The listing builds one solid part. Answer for the finished solid, in the listing's coordinates (mm). Round coordinates to 2 decimals unless told otherwise and drop trailing zeros. Order: outer loops, then holes, each group sorted by start corner. A loop starts at its lowest first (then second) coordinate and runs counter-clockwise, first axis right, second up. Notation, with made-up numbers: (-34, 33) - (0, 33) arc R28 ccw to (0, 70) - close; hole circle Ø8 at (47.25, -19.5). An arc over 180 degrees is marked (long way). One line per item, written item: value. Start each with the question number.
1. Section B-B, the plane y = 0 is taken. Give the vertices of the cut face in (x, z).
2. Section A-A, the plane z = 6.5 is taken. Give the vertices of the cut face in (x, y).
3. Straight lines are drawn through the part: line 1 (Z direction, x = -1.75, y = 1.6); line 2 (Z direction, x = 8, y = -2.55); line 3 (X direction, y = 0, z = 3.5). For each, find the intervals that lie inside material, in ascending order.
4. Flat-ended cylindrical pins translate along their axes: P1, Ø3.5, axis at x = 8, z = 33.5, coming from the -Y side; P2, Ø1.5, axis at y = -2, z = 8.5, coming from the -X side; P3, Ø0.5, axis at y = -2, z = 27.5, coming from the -X side; P4, Ø2.5, axis at x = 8, z = 6.5, coming from the +Y side. Find the tip coordinate at first contact, or state that the pin passes through.
5. Section D-D, the plane z = 21.5 is taken. Give the vertices of the cut face in (x, y), then the cut area to 3 significant figures.
6. Section C-C, the plane x = 8 is taken. Give the vertices of the cut face in (y, z).
from build123d import *

# Parameters (mm, degrees)
ESQUISSE1_R                  = 1.75
BOSS_EXTRU_1_DEPTH           = 40
ENL_V_MAT_EXTRU_3_DEPTH      = 20
ENL_V_MAT_EXTRU_3_DEPTH_BACK = 20
ESQUISSE2_W                  = 17.8
ESQUISSE2_H                  = 8
D_GAGEMENT_M31_D             = 3
D_GAGEMENT_M31_DEPTH         = 10
D_GAGEMENT_M31_CSINK_D       = 4.4
D_GAGEMENT_M31_CSINK_ANGLE   = 90
D_GAGEMENT_M31_TIP           = 0.901290929


with BuildPart() as part:
    # Esquisse1 → Boss.-Extru.1 (new body)
    with BuildSketch(Plane.XY):
        with BuildLine():
            Line((12.5, -1.75), (2.121320344, -1.75))
            ThreePointArc((2.121320344, -1.75), (-1.17260394, 2.487468593), (0, -2.75))
            Line((0, -2.75), (12.5, -2.75))
            Line((12.5, -2.75), (12.5, -1.75))
        make_face()
        Circle(ESQUISSE1_R, mode=Mode.SUBTRACT)
    extrude(amount=BOSS_EXTRU_1_DEPTH)

    # Esquisse2 → Enlèv. mat.-Extru.3 (cut, two sides: drawn at the far end of the back side and taken through both)
    with BuildSketch(Plane(origin=(0, -1.75, 0), x_dir=(1, 0, 0), z_dir=(0, 1, 0)).offset(-ENL_V_MAT_EXTRU_3_DEPTH_BACK)):
        with Locations((-5.3, -12)):
            Rectangle(ESQUISSE2_W, ESQUISSE2_H)
        with Locations((-5.3, -28)):
            Rectangle(ESQUISSE2_W, ESQUISSE2_H)
    extrude(amount=ENL_V_MAT_EXTRU_3_DEPTH + ENL_V_MAT_EXTRU_3_DEPTH_BACK, mode=Mode.SUBTRACT)

    # Dégagement M31
    with Locations(Plane(origin=(0, -1.75, 0), x_dir=(1, 0, 0), z_dir=(0, 1, 0))):
        with Locations((8, -33.5), (8, -6.5)):
            CounterSinkHole(D_GAGEMENT_M31_D / 2, D_GAGEMENT_M31_CSINK_D / 2, depth=D_GAGEMENT_M31_DEPTH, counter_sink_angle=D_GAGEMENT_M31_CSINK_ANGLE)
            with Locations((0, 0, -(D_GAGEMENT_M31_DEPTH + D_GAGEMENT_M31_TIP / 2))):  # 118° drill point
                Cone(0, D_GAGEMENT_M31_D / 2, D_GAGEMENT_M31_TIP, mode=Mode.SUBTRACT)


solid = part.part
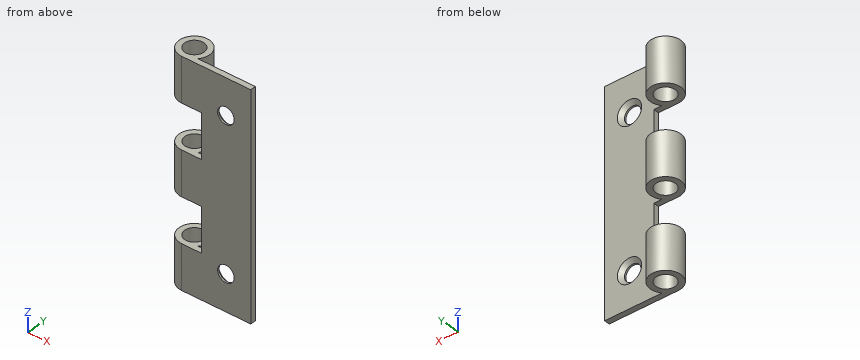
Answer list:
1. outline: (-2.75, 0) - (-1.75, 0) - (-1.75, 8) - (-2.75, 8) - close; (-2.75, 16) - (-1.75, 16) - (-1.75, 24) - (-2.75, 24) - close; (-2.75, 32) - (-1.75, 32) - (-1.75, 40) - (-2.75, 40) - close; (1.75, 0) - (2.75, 0) - (2.75, 8) - (1.75, 8) - close; (1.75, 16) - (2.75, 16) - (2.75, 24) - (1.75, 24) - close; (1.75, 32) - (2.75, 32) - (2.75, 40) - (1.75, 40) - close
2. outline: (0, -2.75) - (6.5, -2.75) - (6.5, -2.45) - (5.8, -1.75) - (2.12, -1.75) arc R2.75 ccw (long way) to start; (9.5, -2.75) - (12.5, -2.75) - (12.5, -1.75) - (10.2, -1.75) - (9.5, -2.45) - close; hole circle Ø3.5 at (0, 0)
3. line 1: z = 0 to 8, 16 to 24, 32 to 40
3. line 2: z = 0 to 5, 8 to 32, 35 to 40
3. line 3: x = -2.75 to -1.75, 1.75 to 2.75
4. P1: stops at y = -2.75
4. P2: stops at x = -2.34
4. P3: stops at x = 3.6
4. P4: passes through
5. outline: (0, -2.75) - (12.5, -2.75) - (12.5, -1.75) - (2.12, -1.75) arc R2.75 ccw (long way) to start; hole circle Ø3.5 at (0, 0)
5. area: 25.2 mm²
6. outline: (-2.75, 0) - (-1.75, 0) - (-1.75, 4.3) - (-2.45, 5) - (-2.75, 5) - close; (-2.75, 8) - (-2.45, 8) - (-1.75, 8.7) - (-1.75, 31.3) - (-2.45, 32) - (-2.75, 32) - close; (-2.75, 35) - (-2.45, 35) - (-1.75, 35.7) - (-1.75, 40) - (-2.75, 40) - close
